from build123d import *

# Parameters (mm, degrees)
SKETCH1_W           = 50
SKETCH1_H           = 50
SKETCH1_W_2         = 44
SKETCH1_H_2         = 44
EXTRUDE_THIN1_DEPTH = 0.75
SKETCH1_3_R         = 1
BOSS_EXTRUDE1_DEPTH = 0.75
SKETCH1_4_W         = 52
SKETCH1_4_H         = 52
SKETCH1_4_W_2       = 50
SKETCH1_4_H_2       = 50
EXTRUDE_THIN2_DEPTH = 2


with BuildPart() as part:
    # Sketch1 → Extrude-Thin1 (new body)
    with BuildSketch(Plane(origin=(0, 0, 0), x_dir=(1, 0, 0), z_dir=(0, 1, 0))):
        with Locations((-6.298946979, 2.1638593)):
            Rectangle(SKETCH1_W, SKETCH1_H)
        with Locations((-6.298946979, 2.1638593)):
            Rectangle(SKETCH1_W_2, SKETCH1_H_2, mode=Mode.SUBTRACT)
    extrude(amount=EXTRUDE_THIN1_DEPTH)

    # Sketch1_3 → Boss-Extrude1 (add)
    with BuildSketch(Plane(origin=(0, 0, 0), x_dir=(1, 0, 0), z_dir=(0, 1, 0))):
        Polygon((-9.430665417, 1.860567093), (-31.298946979, -20.042512046), (-31.298946979, -22.8361407), (-28.435774882, -22.8361407), (-6.59999063, -0.965610581), align=None)
        with Locations((-10.136648367, -1.673842088)):
            Circle(SKETCH1_3_R, mode=Mode.SUBTRACT)
        Polygon((-5.995654771, -0.967859138), (15.907424367, -22.8361407), (18.701053021, -22.8361407), (18.701053021, -19.972968602), (-3.169477097, 1.86281565), align=None)
        with Locations((-2.461245591, -1.673842088)):
            Circle(SKETCH1_3_R, mode=Mode.SUBTRACT)
        Polygon((18.701053021, 27.1638593), (15.837880924, 27.1638593), (-5.997903328, 5.293329182), (-3.167228541, 2.467151508), (18.701053021, 24.370230647), align=None)
        with Locations((-2.461245591, 6.001560689)):
            Circle(SKETCH1_3_R, mode=Mode.SUBTRACT)
        Polygon((-31.298946979, 27.1638593), (-31.298946979, 24.300687203), (-9.428416861, 2.464902951), (-6.602239187, 5.295577739), (-28.505318325, 27.1638593), align=None)
        with Locations((-10.136648367, 6.001560689)):
            Circle(SKETCH1_3_R, mode=Mode.SUBTRACT)
    extrude(amount=BOSS_EXTRUDE1_DEPTH)

    # Sketch1_4 → Extrude-Thin2 (add)
    with BuildSketch(Plane(origin=(0, 0, 0), x_dir=(1, 0, 0), z_dir=(0, 1, 0))):
        with Locations((-6.298946979, 2.1638593)):
            Rectangle(SKETCH1_4_W, SKETCH1_4_H)
        with Locations((-6.298946979, 2.1638593)):
            Rectangle(SKETCH1_4_W_2, SKETCH1_4_H_2, mode=Mode.SUBTRACT)
    extrude(amount=EXTRUDE_THIN2_DEPTH)


solid = part.part
Build history of the part. All positions in model axes, mm. A direction names the side the tool comes from. Round coordinates to 2 decimals unless told otherwise and drop trailing zeros. Order: outer loops, then holes, each group sorted by start corner. A loop starts at its lowest first (then second) coordinate and runs counter-clockwise, first axis right, second up. Notation, with made-up numbers: M 57.5,34 L 85.5,34 A19 ccw 85.5,40 Z; hole C 47.25,41.25 d3. An arc over 180 degrees is marked long. Use CSV: the item, a comma, the result in double quotes. Start each with the question number.
(1) Mould opens along X. For faces 1 (the face through (-2.68, 0.37, 2.65)), 2 (the face through (-32.299, 1, -2)), 3 (the face through (-7, 1, -28.164)) say: +X half, -X half, draft (parallel to the pull), parting line (faces both ways), or undercut.
(2) Tool access for faces 4 (the face through (-31.299, 1, -2)), 5 (the face through (-16.15, 0.37, 10.53)): list every direction of +Z, -Z, +X, -X, +Y, -Y with a clear straight run to the whole face (end or side of a thin tool).
(3) Flat gauge pins, fed straight in: P1, Ø5, axis at x = 8.5, z = 13, coming from the +Y side; P2, Ø6, axis at x = -13.5, z = -12.5, coming from the -Y side. Where does each tip first touch, or does it go through?
(4) Cut at A-A on x = -23.5. List the corners of the cut face in (y, z).
(5) Cut at B-B on y = 1.3. List the corners of the cut face in (x, z), then the cut area to 3 significant figures.
(6) Drill centre lines: probe 1 along Z at (x, y) = (-3.5, 1.1); probe 2 along X at (y, z) = (1.55, 4.5); probe 3 along X at (y, z) = (0.2, -14). Where is each one in solid material? Low to high.
(7) Cut at C-C on z = 9. List the corners of the cut face in (x, y).
Findings:
1,face 1,"undercut"
1,face 2,"-X half"
1,face 3,"draft"
2,face 4,"+Y"
2,face 5,"+Y, -Y"
3,P1,"stops at y = 0.75"
3,P2,"stops at y = 0"
4,outline,"M 0,-28.16 L 2,-28.16 L 2,-27.16 L 0.75,-27.16 L 0.75,-24.16 L 0,-24.16 Z; M 0,-22.17 L 0.75,-22.17 L 0.75,-16.51 L 0,-16.51 Z; M 0,12.23 L 0.75,12.23 L 0.75,17.89 L 0,17.89 Z; M 0,19.84 L 0.75,19.84 L 0.75,22.84 L 2,22.84 L 2,23.84 L 0,23.84 Z"
5,outline,"M -32.3,-28.16 L 19.7,-28.16 L 19.7,23.84 L -32.3,23.84 Z; hole M -31.3,-27.16 L 18.7,-27.16 L 18.7,22.84 L -31.3,22.84 Z"
5,area,"204 mm^2"
6,probe 1,"z = -28.16 to -27.16, 22.84 to 23.84"
6,probe 2,"x = -32.3 to -31.3, 18.7 to 19.7"
6,probe 3,"x = -32.3 to -28.3, -20.98 to -15.32, 2.69 to 8.35, 15.7 to 19.7"
7,outline,"M -32.3,0 L -28.3,0 L -28.3,0.75 L -31.3,0.75 L -31.3,2 L -32.3,2 Z; M -20.27,0 L -14.62,0 L -14.62,0.75 L -20.27,0.75 Z; M 2.05,0 L 7.71,0 L 7.71,0.75 L 2.05,0.75 Z; M 15.7,0 L 19.7,0 L 19.7,2 L 18.7,2 L 18.7,0.75 L 15.7,0.75 Z"
